For this review, use the dimensioned drawing (mm, ordinates from the lowest corner) and the shaded views. Round coordinates to 2 decimals unless told otherwise and drop trailing zeros. Order: outer loops, then holes, each group sorted by start corner. A loop starts at its lowest first (then second) coordinate and runs counter-clockwise, first axis right, second up. Notation, with made-up numbers: (-22, 75.25) -> (5, 75.25) arc R35 ccw to (5, 114.25) -> close; hole circle Ø6 at (4.25, 65.25). An arc over 180 degrees is marked (long way). Answer in a Markdown table with one row per item.
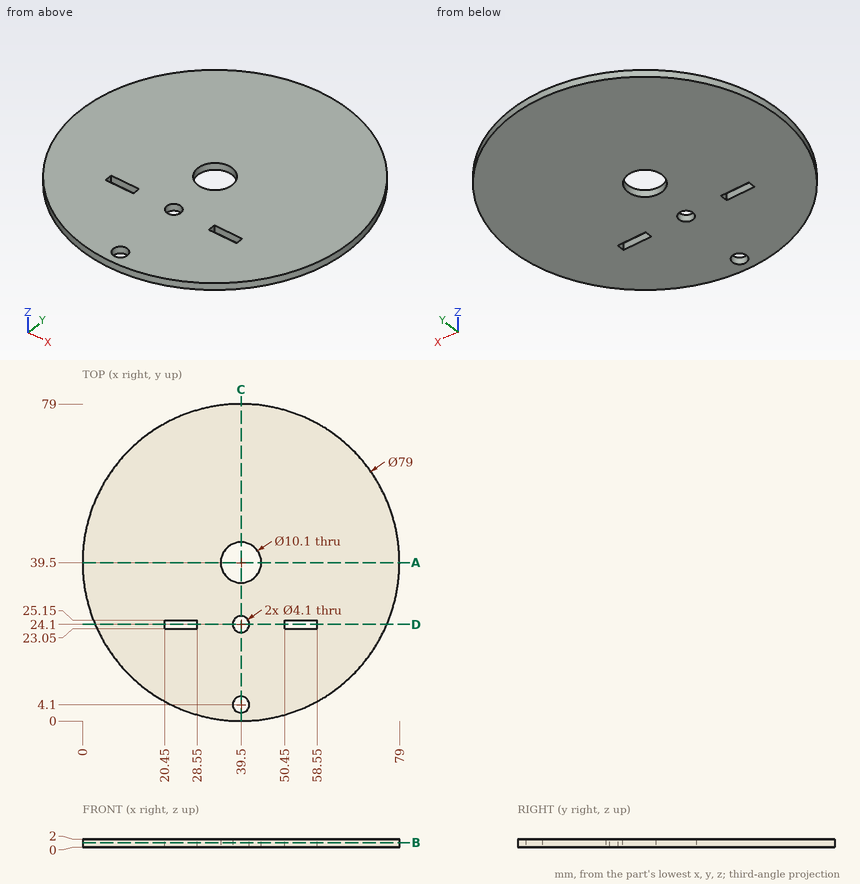
Q1. Take a section at B-B, the plane z = 1.1. Write out the cut boundary in (x, y), then the cut area to 3 significant figures.
Answer key:
| item | result |
|---|---|
| outline | circle Ø79 at (39.5, 39.5); hole (20.45, 23.05) -> (28.55, 23.05) -> (28.55, 25.15) -> (20.45, 25.15) -> close; hole circle Ø10.1 at (39.5, 39.5); hole circle Ø4.1 at (39.5, 4.1); hole circle Ø4.1 at (39.5, 24.1); hole (50.45, 23.05) -> (58.55, 23.05) -> (58.55, 25.15) -> (50.45, 25.15) -> close |
| area | 4,760 mm^2 |
Q2. Take a section at D-D, the plane y = 24.1. Write out the cut boundary in (x, z).
Answer key:
| item | result |
|---|---|
| outline | (3.13, 0) -> (20.45, 0) -> (20.45, 2) -> (3.13, 2) -> close; (28.55, 0) -> (37.45, 0) -> (37.45, 2) -> (28.55, 2) -> close; (41.55, 0) -> (50.45, 0) -> (50.45, 2) -> (41.55, 2) -> close; (58.55, 0) -> (75.87, 0) -> (75.87, 2) -> (58.55, 2) -> close |
Q3. Take a section at A-A, the plane y = 39.5. Write out the cut boundary in (x, z).
Answer key:
| item | result |
|---|---|
| outline | (0, 0) -> (34.45, 0) -> (34.45, 2) -> (0, 2) -> close; (44.55, 0) -> (79, 0) -> (79, 2) -> (44.55, 2) -> close |
Q4. Clearance check with flat-ended pins moving along their axes: pin 1 Ø4.5 at (x, y) = (39.5, 24.1) entering from +Z; pin 2 Ø1 at (y, z) = (24, 1.5) entering from -X. State where each tip first meets the part, or that it passes through.
Answer key:
| item | result |
|---|---|
| pin 1 | stops at z = 2 |
| pin 2 | stops at x = 2.96 |
Q5. To check wall thickness, follow probe 1 along Y at (x, z) = (39.5, 0.55); probe 2 along Y at (x, z) = (41, 1.55); probe 3 along Y at (x, z) = (21, 0.4). State the ranges of each line that lie inside material, in increasing order.
Answer key:
| item | result |
|---|---|
| probe 1 | y = 0 to 2.05, 6.15 to 22.05, 26.15 to 34.45, 44.55 to 79 |
| probe 2 | y = 0.03 to 2.7, 5.5 to 22.7, 25.5 to 34.68, 44.32 to 78.97 |
| probe 3 | y = 4.6 to 23.05, 25.15 to 74.4 |
Q6. Take a section at C-C, the plane x = 39.5. Write out the cut boundary in (y, z).
Answer key:
| item | result |
|---|---|
| outline | (0, 0) -> (2.05, 0) -> (2.05, 2) -> (0, 2) -> close; (6.15, 0) -> (22.05, 0) -> (22.05, 2) -> (6.15, 2) -> close; (26.15, 0) -> (34.45, 0) -> (34.45, 2) -> (26.15, 2) -> close; (44.55, 0) -> (79, 0) -> (79, 2) -> (44.55, 2) -> close |
